from build123d import *

# Parameters (mm, degrees)
F0_W      = 50.8
F0_H      = 50.8
F1_DEPTH  = 50.8
F2_W      = 101.6
F2_H      = 101.6
F3_DEPTH  = 76.2
F3_FACE_W = 101.6
F3_FACE_H = 101.6
F4_DEPTH  = 25.4
F6_D      = 25.4
F8_D      = 25.4
F10_D     = 25.4


with BuildPart() as f1:
    # F0 (on Front) → F1 (new body)
    with BuildSketch(Plane.XZ):
        with Locations((-25.4, 25.4)):
            Rectangle(F0_W, F0_H)
    extrude(amount=F1_DEPTH)

    # F2 (on Front) → F3 (join)
    with BuildSketch(Plane.XZ):
        with Locations((-25.4, 25.4)):
            Rectangle(F2_W, F2_H)
    extrude(amount=F3_DEPTH)

    # F3_face (on face) → F4 (join)
    with BuildSketch(Plane(origin=(-25.4, 0, 25.4), x_dir=(1, 0, 0), z_dir=(0, 1, 0))):
        Rectangle(F3_FACE_W, F3_FACE_H)
    extrude(amount=F4_DEPTH)

    # F6 (through all)
    with Locations(Plane.XY.offset(76.2)):
        with Locations((-25.4, -25.4)):
            Hole(F6_D / 2)

    # F8 (through all)
    with Locations(Plane(origin=(-76.2, 0, 0), x_dir=(0, -1, 0), z_dir=(-1, 0, 0))):
        with Locations((25.4, 25.4)):
            Hole(F8_D / 2)

    # F10 (through all)
    with Locations(Plane.XZ.offset(76.2)):
        with Locations((-25.4, 25.4)):
            Hole(F10_D / 2)


solid = f1.part
For this review, take the finished solid that the model builds, in its own axes (mm). Give positions to 0.01 mm unless a question says otherwise; leave off trailing zeros. Loops run counter-clockwise (first coordinate to the right, second up) from the corner with the lowest first, then second, coordinate; pieces in that order, holes last. Notation, with made-up numbers: M 65.25,79 L 88.25,79 A23 cw 88.25,115 Z; hole C 83,-25.75 d2. An arc over 180 degrees is marked long. Answer as a JSON object with one key per item and string values. Group by question number.
Q1. Insertion check: P1, Ø6, axis at y = -33, z = 21, coming from the +X side. The pin has a flat end and moves straight along its axis. Give the tip position at first contact, or say it passes through.
Q2. Mouldability with a two-part tool opening along X and no side actions: class faces 1 (the cylindrical face through (-12.712, -24.842, -4.783)), 2 (the flat face through (-76.2, -37, 37)), 3 (the cylindrical face through (-12.712, 4.783, 25.958)), 4 (the flat face through (-37, -37, -25.4)) as +X half, -X half, draft (parallel to the pull), parting line (faces both ways), or undercut.
Q3. Add section C-C on z = 2. Give the boundary of the cut face in (x, y).
Q4. For probe 1 along Y at (x, z) = (-43, 25); probe 2 along X at (y, z) = (-25.4, -16); probe 3 along Z at (x, y) = (-53, -25), list the stretches that pass through material, from the lowest coordinate up. Write a range as [from, to].
Q5. Add section A-A on y = -25.4. Give the boundary of the cut face in (x, z), and give its area (3 significant figures).
Q6. Add section D-D on y = -40.5. Give the boundary of the cut face in (x, z), and give its area (3 significant figures).
Checked values:
{
 "1": {"P1": "through"},
 "2": {"face 1": "undercut", "face 2": "-X half", "face 3": "undercut", "face 4": "draft"},
 "3": {"outline": "M -76.2,-76.2 L 25.4,-76.2 L 25.4,25.4 L -76.2,25.4 Z; hole C -25.4,-25.4 d25.4"},
 "4": {"probe 1": "[-76.2, -38.09], [-12.71, 25.4]", "probe 2": "[-76.2, -38.1], [-12.7, 25.4]", "probe 3": "[-25.4, 12.71], [38.09, 76.2]"},
 "5": {"outline": "M -76.2,-25.4 L -38.1,-25.4 L -38.1,12.7 L -76.2,12.7 Z; M -76.2,38.1 L -38.1,38.1 L -38.1,76.2 L -76.2,76.2 Z; M -12.7,-25.4 L 25.4,-25.4 L 25.4,12.7 L -12.7,12.7 Z; M -12.7,38.1 L 25.4,38.1 L 25.4,76.2 L -12.7,76.2 Z", "area": "5,810 mm²"},
 "6": {"outline": "M -76.2,-25.4 L 25.4,-25.4 L 25.4,76.2 L -76.2,76.2 Z; hole C -25.4,25.4 d25.4", "area": "9,820 mm²"}
}
